The model under review builds one solid part; all positions refer to its coordinate system, in mm. A direction names the side the tool comes from. Give positions to 0.01 mm unless a question says otherwise; leave off trailing zeros. Write each loop counter-clockwise with the first axis right and the second up, starting at its lowest first coordinate (ties: lowest second). Pieces come first, ordered by that corner, then holes. Notation, with made-up numbers: (0, 86) - (35, 86) arc R16 cw to (35, 90) - close; hole circle Ø4 at (-10.75, 35). An arc over 180 degrees is marked (long way). Write item = value, one per line.
Autodesk Inventor part; units mm, degrees
ref_plane "YZ Plane" through (0, 0, 0) normal (1, 0, 0) x (0, 1, 0)
ref_plane "XZ Plane" through (0, 0, 0) normal (0, 1, 0) x (-1, 0, 0)
ref_plane "XY Plane" through (0, 0, 0) normal (0, 0, 1) x (1, 0, 0)
sketch "Sketch2" plane through (0, 0, 0) normal (0, 1, 0) x (-1, 0, 0)
  line L0 (-22, 25.4) -> (22, 25.4)
  line L1 (22, 25.4) -> (22, -25.4)
  line L2 (22, -25.4) -> (-22, -25.4)
  line L3 (-22, -25.4) -> (-22, 25.4)
  line L4 (-22, 25.4) -> (22, -25.4) construction
  line L5 (22, 25.4) -> (-22, -25.4) construction
  point P0 (0, 0)
  dimension "d0" = 50.8
  dimension "d1" = 44
extrude "Extrusion1" add sketch "Sketch2" along normal blind 25.4
sketch "Sketch3" plane through (-22, 0, 25.4) normal (0, 0, 1) x (1, 0, 0)
  line L0 (0, 25.4) -> (44, 25.4) construction
  line L1 (0, 0) -> (44, 0) construction
  line L2 (44, 0) -> (44, 25.4) construction
  line L3 (44, 25.4) -> (0, 25.4) construction
  line L4 (0, 25.4) -> (0, 0) construction
  line L5 (0, 0) -> (44, 25.4) construction
  line L6 (44, 0) -> (0, 25.4) construction
  point P0 (22, 0)
  point P1 (22, 12.7)
hole "Hole1" at (0, 12.7, 25.4) direction (0, 0, -1) diameter 4.134 depth 19.05 tip angle 118
mirror "Mirror1" about plane through (0, 0, 0) normal (0, 0, 1) of "Hole1"
sketch "Sketch4" plane through (0, 25.4, 0) normal (0, 1, 0) x (1, 0, 0)
  line L0 (10, -7.5) -> (10, 7.5) construction
  line L1 (10, 7.5) -> (-10, 7.5) construction
  line L2 (-10, 7.5) -> (-10, -7.5) construction
  line L3 (-10, -7.5) -> (10, -7.5) construction
  line L4 (10, -7.5) -> (-10, 7.5) construction
  line L5 (10, 7.5) -> (-10, -7.5) construction
  circle A0 centre (-10, 7.5) radius 3
  circle A1 centre (10, 7.5) radius 3
  circle A2 centre (10, -7.5) radius 3
  circle A3 centre (-10, -7.5) radius 3
  point P0 (0, 0)
  dimension "d15" = 20
  dimension "d16" = 15
  dimension "d14" = 6
  dimension "d13" = 6
  dimension "d12" = 6
  dimension "d11" = 6
extrude "Extrusion2" cut sketch "Sketch4" against normal blind 5
sketch "Sketch5" plane through (-10, 20.4, 7.5) normal (0, 1, 0) x (1, 0, 0)
  circle A0 centre (0, 15) radius 3
  circle A1 centre (20, 0) radius 3
  circle A2 centre (20, 15) radius 3
  point P0 (16, 18)
  point P1 (0, 0)
hole "Hole2" at (-10, 20.4, -7.5) at (-10, 20.4, 7.5) at (10, 20.4, 7.5) at (10, 20.4, -7.5) direction (0, -1, 0) diameter 3.5 end through all
properties part number "Mass 2" material "Steel, Mild"
1. Take a section at C-C on y = 8.25. Give the boundary of the cut face in (x, z), and give its area (3 significant figures).
Findings below:
outline = (-22, -25.4) - (22, -25.4) - (22, 25.4) - (-22, 25.4) - close; hole circle Ø3.5 at (-10, -7.5); hole circle Ø3.5 at (-10, 7.5); hole circle Ø3.5 at (10, -7.5); hole circle Ø3.5 at (10, 7.5)
area = 2,200 mm²
2. Take a section at B-B on x = -10. Give the boundary of the cut face in (y, z).
Findings below:
outline = (0, -25.4) - (25.4, -25.4) - (25.4, -10.5) - (20.4, -10.5) - (20.4, -9.25) - (0, -9.25) - close; (0, -5.75) - (20.4, -5.75) - (20.4, -4.5) - (25.4, -4.5) - (25.4, 4.5) - (20.4, 4.5) - (20.4, 5.75) - (0, 5.75) - close; (0, 9.25) - (20.4, 9.25) - (20.4, 10.5) - (25.4, 10.5) - (25.4, 25.4) - (0, 25.4) - close
3. For line 1 (X direction, y = 6.5, z = -7.5); line 2 (X direction, y = 22.3, z = -7.5); line 3 (Z direction, x = 10, y = 22.8), list the stretches that pass through material, from the lowest coordinate up. Write a range as from..to.
Findings below:
line_1 = -22..-11.75, -8.25..8.25, 11.75..22
line_2 = -22..-13, -7..7, 13..22
line_3 = -25.4..-10.5, -4.5..4.5, 10.5..25.4
4. Draft analysis for pull direction X (two halves, no side actions). For faces 3 (the flat face through (-22, 13, 0)), 4 (the cylindrical face through (-0.79, 10.79, -15.74)), 5 (the flat face through (0, 15, -25.4)), state which applies: +X half, -X half, draft (parallel to the pull), parting line (faces both ways), or undercut.
Findings below:
face_3 = -X half
face_4 = undercut
face_5 = draft
5. Take a section at D-D on y = 22. Give the boundary of the cut face in (x, z), and give its area (3 significant figures).
Findings below:
outline = (-22, -25.4) - (22, -25.4) - (22, 25.4) - (-22, 25.4) - close; hole circle Ø6 at (-10, -7.5); hole circle Ø6 at (-10, 7.5); hole circle Ø6 at (10, -7.5); hole circle Ø6 at (10, 7.5)
area = 2,120 mm²
6. Take a section at A-A on z = 7.5. Give the boundary of the cut face in (x, y), and give its area (3 significant figures).
Findings below:
outline = (-22, 0) - (-11.75, 0) - (-11.75, 20.4) - (-13, 20.4) - (-13, 25.4) - (-22, 25.4) - close; (-8.25, 0) - (8.25, 0) - (8.25, 20.4) - (7, 20.4) - (7, 25.4) - (-7, 25.4) - (-7, 20.4) - (-8.25, 20.4) - close; (11.75, 0) - (22, 0) - (22, 25.4) - (13, 25.4) - (13, 20.4) - (11.75, 20.4) - close; hole circle Ø4.13 at (0, 12.7)
area = 901 mm²
7. Insertion check: P1, Ø5, axis at x = -10, z = -7.5, coming from the +Y side; P2, Ø3, axis at x = 10, z = -7.5, coming from the +Y side. Each pin has a flat end and moves straight along its axis. Give the tip position at first contact, or say it passes through.
Findings below:
P1 = 20.4
P2 = through
8. Machinability: for faces 1 (the flat face through (12, 20.4, -8)), 2 (the cylindrical face through (8.5, 10.1, 8.4)), which of the approach directions +Z, -Z, +X, -X, +Y, -Y give a long, thin tool a straight path to every point of the face, cutting with its end or side? Answer none if there is none.
Findings below:
face_1 = +Y
face_2 = +Y, -Y
